For this review, take the finished solid that the model builds, in its own axes (mm). Coordinates: 2 decimals unless noted, no trailing zeros. Order: outer loops, then holes, each group sorted by start corner. A loop starts at its lowest first (then second) coordinate and runs counter-clockwise, first axis right, second up. Notation, with made-up numbers: (31, 77) -> (87, 77) arc R14 cw to (87, 98) -> close; hole circle Ø2 at (22.25, 2.25). An arc over 180 degrees is marked (long way). Answer as a JSON object with one key per item and string values. Group by question number.
1) Add section D-D, the plane y = 17.5. Write out the cut boundary in (x, z).
2) Wall thickness on L1, parallel to X at y = -1.5, z = 2.25; L2, parallel to X at y = 4, z = 0.95; L3, parallel to Y at x = -5.5, z = 2.55: over which ranges is each line inside the solid? List them lowest first.
3) Add section A-A, the plane y = -38. Write out the cut boundary in (x, z).
4) For pin 1 (1.5 mm diameter, centred on y = 33.5, z = 2.5, fed in from +X); pin 2 (10.5 mm diameter, centred on x = 20.95, y = -12.09, fed in from -Z), all flat-tipped, find the tip position at first contact; note any pin that passes through.
5) Add section C-C, the plane z = 0.7. Count the separate pieces of the cut face and the enclosed holes in it, then the cut area to 3 significant figures.
6) Add section B-B, the plane x = 0. Write out the cut boundary in (y, z).
from build123d import *

# Parameters (mm, degrees)
F0_R     = 10
F0_R_2   = 4.58
F0_R_3   = 11
F1_DEPTH = 3


with BuildPart() as f1:
    # F0 (on Top) → F1 (new body)
    with BuildSketch(Plane.XY):
        with BuildLine():
            Line((-10.977667, 20.721382), (-6.590549, 13.474593))
            ThreePointArc((-6.590549, 13.474593), (-12.927762, 7.607429), (-14.979629, -0.781476))
            Line((-14.979629, -0.781476), (-27.635152, -1.044408))
            Line((-27.635152, -1.044408), (-33.859359, -12.361615))
            Line((-33.859359, -12.361615), (-29.160745, -20.122942))
            Line((-29.160745, -20.122942), (-36.160002, -33.056272))
            Line((-36.160002, -33.056272), (-27.966558, -46.385655))
            Line((-27.966558, -46.385655), (-12.326252, -45.954617))
            Line((-12.326252, -45.954617), (-4.879389, -32.194194))
            Line((-4.879389, -32.194194), (-12.45641, -19.867629))
            Line((-12.45641, -19.867629), (-8.374066, -12.444879))
            ThreePointArc((-8.374066, -12.444879), (-0.124346, -14.999485), (8.166593, -12.582001))
            Line((8.166593, -12.582001), (14.72206, -23.41054))
            Line((14.72206, -23.41054), (27.635152, -23.142257))
            Line((27.635152, -23.142257), (32.007352, -15.192475))
            Line((32.007352, -15.192475), (46.707572, -14.787345))
            Line((46.707572, -14.787345), (54.154435, -1.026922))
            Line((54.154435, -1.026922), (45.960991, 12.302461))
            Line((45.960991, 12.302461), (30.320685, 11.871423))
            Line((30.320685, 11.871423), (23.434076, -0.853753))
            Line((23.434076, -0.853753), (14.964615, -1.029714))
            ThreePointArc((14.964615, -1.029714), (13.052108, 7.392056), (6.813036, 13.363478))
            Line((6.813036, 13.363478), (12.913093, 24.454948))
            Line((12.913093, 24.454948), (6.224207, 35.503873))
            Line((6.224207, 35.503873), (-2.846607, 35.315417))
            Line((-2.846607, 35.315417), (-10.54757, 47.843616))
            Line((-10.54757, 47.843616), (-26.187877, 47.412578))
            Line((-26.187877, 47.412578), (-33.63474, 33.652155))
            Line((-33.63474, 33.652155), (-25.441296, 20.322772))
            Line((-25.441296, 20.322772), (-10.977667, 20.721382))
        make_face()
        with Locations((-20.519695, -32.625233)):
            Circle(F0_R, mode=Mode.SUBTRACT)
        with Locations((-20.946266, -12.093333)):
            Circle(F0_R_2, mode=Mode.SUBTRACT)
        Circle(F0_R_3, mode=Mode.SUBTRACT)
        with Locations((20.946266, -12.093333)):
            Circle(F0_R_2, mode=Mode.SUBTRACT)
        with Locations((38.514128, -1.457961)):
            Circle(F0_R, mode=Mode.SUBTRACT)
        with Locations((0, 24.186665)):
            Circle(F0_R_2, mode=Mode.SUBTRACT)
        with Locations((-17.994433, 34.083194)):
            Circle(F0_R, mode=Mode.SUBTRACT)
    extrude(amount=F1_DEPTH)


solid = f1.part
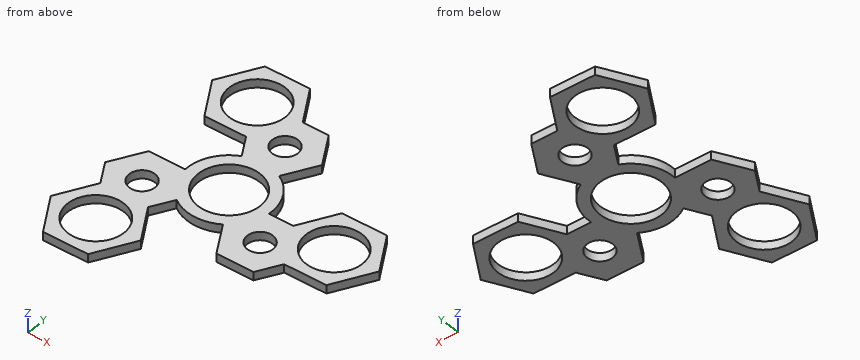
Output values:
{
 "1": {"outline": "(-9.03, 0) -> (9.09, 0) -> (9.09, 3) -> (-9.03, 3) -> close"},
 "2": {"L1": "x = -27.89 to -10.9, 10.9 to 28.51, 48.51 to 53.9", "L2": "x = -14.46 to -10.25, 10.25 to 14.46, 26.06 to 30.13, 46.89 to 51.06", "L3": "y = -33.34 to -31.18, -13.96 to -9.53, 9.53 to 39.63"},
 "3": {"outline": "(-33.12, 0) -> (-28.95, 0) -> (-28.95, 3) -> (-33.12, 3) -> close; (-12.09, 0) -> (-8.02, 0) -> (-8.02, 3) -> (-12.09, 3) -> close"},
 "4": {"pin 1": "stops at x = 7.89", "pin 2": "stops at z = 0"},
 "5": {"separate pieces": "1", "enclosed holes": "7", "area": "2,150 mm²"},
 "6": {"outline": "(-15, 0) -> (-11, 0) -> (-11, 3) -> (-15, 3) -> close; (11, 0) -> (19.61, 0) -> (19.61, 3) -> (11, 3) -> close; (28.77, 0) -> (35.37, 0) -> (35.37, 3) -> (28.77, 3) -> close"}
}
